The listing builds one solid part. Answer for the finished solid, in the listing's coordinates (mm). A direction names the side the tool comes from. Give positions to 0.01 mm unless a question says otherwise; leave off trailing zeros. Order: outer loops, then holes, each group sorted by start corner. A loop starts at its lowest first (then second) coordinate and runs counter-clockwise, first axis right, second up.
```python
from build123d import *

# Parameters (mm, degrees)
F0_R     = 15.010998
F1_DEPTH = 40
F2_R     = 2.587431
F3_DEPTH = 5
F4_R     = 7.580978
F5_DEPTH = 10
F6_R     = 5.08


with BuildPart() as f1:
    # F0 (on Front) → F1 (new body)
    with BuildSketch(Plane.XZ):
        with Locations((0.77934, -14.990753)):
            Circle(F0_R)
    extrude(amount=F1_DEPTH)

    # F2 (on face) → F3 (cut)
    with BuildSketch(Plane(origin=(0, 0, 0), x_dir=(-1, 0, 0), z_dir=(0, 1, 0))):
        with Locations((-0.003086, -4.838753)):
            Circle(F2_R)
    extrude(amount=-F3_DEPTH, mode=Mode.SUBTRACT)

    # F4 (on face) → F5 (join)
    with BuildSketch(Plane.XZ.offset(40)):
        with Locations((0.77934, -14.990753)):
            Circle(F4_R)
    extrude(amount=F5_DEPTH)

    # F6
    f6_edges = [f1.edges().sort_by_distance(p)[0] for p in [
        (-6.801638, -50, -14.990753),
    ]]
    fillet(f6_edges, radius=F6_R)


solid = f1.part
```
1) For a pull along X with two mould halves and no side action, classify faces 4 (the flat face through (1, 0, -15)), 5 (the flat face through (0, -5, -5)), 6 (the cylindrical face through (-2.475, -19.72, -29.645)) as +X half, -X half, draft (parallel to the pull), parting line (faces both ways), or undercut.
Geometry says:
face 4: draft
face 5: undercut
face 6: parting line
2) Straight lines are drawn through the part: probe 1 along Z at (x, y) = (1, -36.5); probe 2 along Y at (x, z) = (11.5, -22); probe 3 along X at (y, z) = (-11.5, -15.5). For each, find the intervals that lie inside material, in ascending order.
Geometry says:
probe 1: z = -30 to 0.02
probe 2: y = -40 to 0
probe 3: x = -14.22 to 15.78
3) Given P1, Ø1, axis at x = -2.5, y = -27.5, coming from the -Z side; P2, Ø4, axis at x = 9.5, y = -44.5, coming from the -Z side; P3, Ø4, axis at x = 4.5, y = -23.5, coming from the -Z side, each flat-ended and moving along its own axis, determine where each tip first touches the part or whether it passes through.
Geometry says:
P1: stops at z = -29.74
P2: stops at z = -18.5
P3: stops at z = -29.9
4) Find section A-A (z = -6.5). Write down the section's boundary in (x, y), then the cut area to 3 significant figures.
Geometry says:
outline: (-11.6, -40) - (13.16, -40) - (13.16, 0) - (1.99, 0) - (1.99, -5) - (-1.98, -5) - (-1.98, 0) - (-11.6, 0) - close
area: 970 mm2
5) Find section B-B (y = -41). Write down the section's boundary in (x, z).
Geometry says:
outline: circle Ø15.16 at (0.78, -14.99)
6) Find section C-C (x = 13). Write down the section's boundary in (y, z), then the cut area to 3 significant figures.
Geometry says:
outline: (-40, -23.71) - (0, -23.71) - (0, -6.27) - (-40, -6.27) - close
area: 697 mm2
7) A tool of negligible diameter and unlimited length cuts with its end or side. For faces 1 (the flat face through (-6, -40, -11)), 2 (the flat face through (1, -50, -15)), 3 (the cylindrical face through (-1.191, -2.465, -7.134)), from which of +Z, -Z, +X, -X, +Y, -Y can it reach the whole face along a straight path? Write none if from no direction.
Geometry says:
face 1: -Y
face 2: +Z, -Z, +X, -X, -Y
face 3: +Y
8) Find section D-D (z = -24). Write down the section's boundary in (x, y).
Geometry says:
outline: (-11.23, -40) - (12.79, -40) - (12.79, 0) - (-11.23, 0) - close
